Check sheet for the drawn part. Datum: minimum x, y, z corner. Units: mm. Give positions to 0.01 mm unless a question says otherwise; leave off trailing zeros. Write each loop counter-clockwise with the first axis right and the second up, starting at its lowest first coordinate (ties: lowest second). Pieces come first, ordered by that corner, then holes. Notation, with made-up numbers: (-5.75, 4) - (24.25, 4) arc R36 ccw to (24.25, 40) - close; hole circle Ø7 at (-37, -15). An arc over 180 degrees is marked (long way). Answer as a JSON object with one key per item and string values. Group by question number.
Item 1: Go/stop test with flat-tipped pins: pin 1 (0.8 mm diameter, centred on y = 0.5, z = 13, fed in from +X) (3 decimals); pin 2 (0.8 mm diameter, centred on x = 1, y = 2, fed in from +Z); pin 3 (1.4 mm diameter, centred on x = 0.5, y = 1.5, fed in from -Z); pin 4 (12 mm diameter, centred on x = 34.5, z = 33.5, fed in from -Y). Record where each tip stops, or that it passes through.
Item 2: Scan line: line 1 along X through (y, z) = (2.5, 28.5) (1 decimal). Record every from-to range of solid material in increasing order. Write a range as [from, to].
Item 3: Sectioned sample at B-B, the plane z = 13.5. Record the boundary of the cut face in (x, y) (1 decimal), and give its area (3 significant figures).
Item 4: Sectioned sample at A-A, the plane y = 1.8. Record the boundary of the cut face in (x, z) (1 decimal), and give its area (3 significant figures).
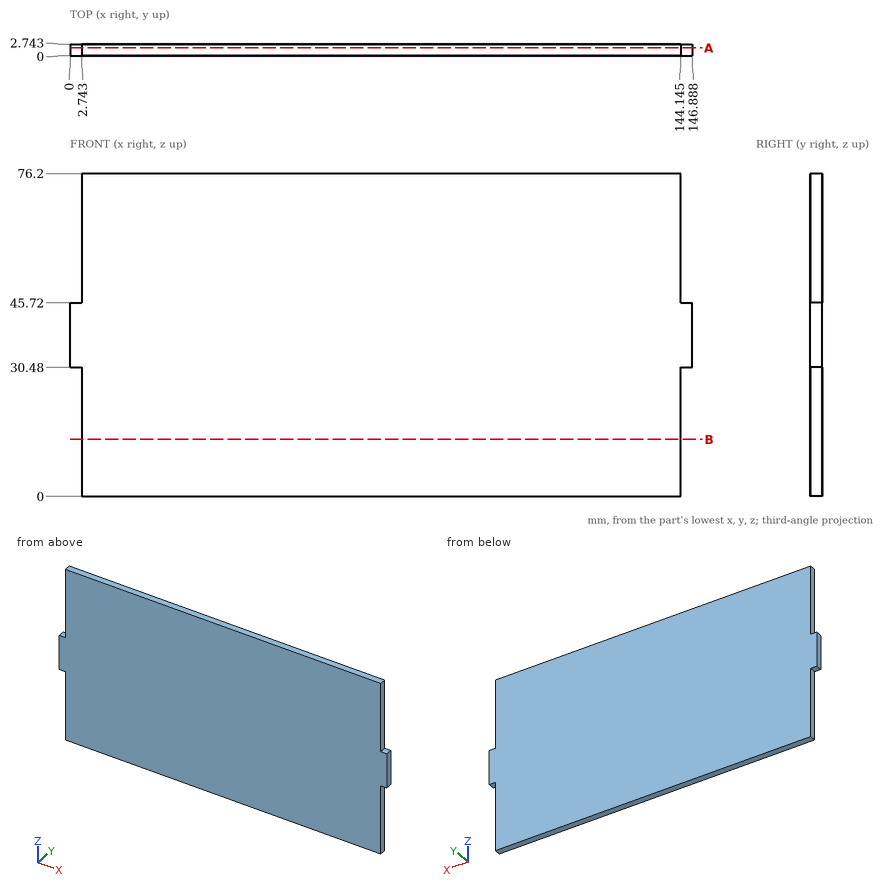
Geometry check:
{
 "1": {"pin 1": "x = 144.145", "pin 2": "z = 45.72", "pin 3": "z = 30.48", "pin 4": "y = 0"},
 "2": {"line 1": "[2.7, 144.1]"},
 "3": {"outline": "(2.7, 0) - (144.1, 0) - (144.1, 2.7) - (2.7, 2.7) - close", "area": "388 mm^2"},
 "4": {"outline": "(0, 30.5) - (2.7, 30.5) - (2.7, 0) - (144.1, 0) - (144.1, 30.5) - (146.9, 30.5) - (146.9, 45.7) - (144.1, 45.7) - (144.1, 76.2) - (2.7, 76.2) - (2.7, 45.7) - (0, 45.7) - close", "area": "10,900 mm^2"}
}
